Design review of the part built by this model. Coordinates are the model's own, in mm. Face numbers are marked on the shaded views. A direction names the side the tool comes from. Coordinates: 2 decimals unless noted, no trailing zeros. Write each loop counter-clockwise with the first axis right and the second up, starting at its lowest first coordinate (ties: lowest second). Pieces come first, ordered by that corner, then holes.
Q1. Insertion check: pin 1 (4 mm diameter, centred on x = -7, z = -7.5, fed in from +Y); pin 2 (1 mm diameter, centred on x = -11.5, z = -11.5, fed in from +Y); pin 3 (1.7 mm diameter, centred on x = 0, z = 0.5, fed in from +Y). Each pin has a flat end and moves straight along its axis. Give the tip position at first contact, or say it passes through.
Q2. For probe 1 along X at (y, z) = (23.75, 11.43) (3 decimals); probe 2 along X at (y, z) = (8, -0.25); probe 3 along Z at (x, y) = (-0.5, 23), list the stretches that pass through material, from the lowest coordinate up.
Q3. Take a section at A-A (y = 4). Give the boundary of the cut face in (x, z) (1 decimal).
Q4. Mouldability with a two-part tool opening along Z and no side actions: class the marked faces 3, 4 and 5 as pulls with the +Z half, pulls with the -Z half, needs draft (parallel to the pull), parting line crosses it, or undercut.
Q5. Take a section at D-D (y = 21.5). Give the boundary of the cut face in (x, z) (3 decimals).
Q6. Take a section at B-B (z = 9.5). Give the boundary of the cut face in (x, y).
Q7. Machinability: for the marked faces 1 and 2, which of the approach directions +Z, -Z, +X, -X, +Y, -Y give a long, thin tool a straight path to every point of the face, cutting with its end or side? Answer none if there is none.
Q8. Take a section at C-C (x = -11.43). Give the boundary of the cut face in (y, z) (3 decimals), and give its area (3 significant figures).
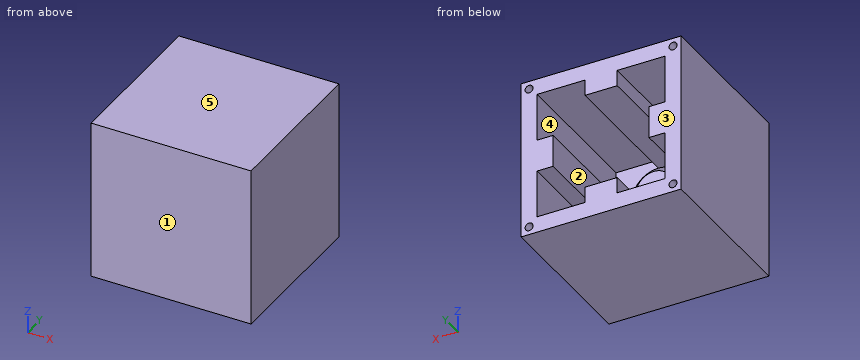
```python
from build123d import *

# Parameters (mm, degrees)
SKETCH1_W           = 25.4
SKETCH1_H           = 25.4
BOSS_EXTRUDE1_DEPTH = 25.4
CUT_EXTRUDE2_DEPTH  = 22.86
SKETCH4_R           = 0.635
CUT_EXTRUDE4_DEPTH  = 7.62
SKETCH5_R           = 4.1275
BOSS_EXTRUDE2_DEPTH = 7.62
CHAMFER1_SIZE       = 1.27


with BuildPart() as part:
    # Sketch1 → Boss-Extrude1 (new body)
    with BuildSketch(Plane(origin=(0, 0, 0), x_dir=(1, 0, 0), z_dir=(0, 1, 0))):
        Rectangle(SKETCH1_W, SKETCH1_H)
    extrude(amount=BOSS_EXTRUDE1_DEPTH)

    # Sketch3 → Cut-Extrude2 (cut)
    with BuildSketch(Plane(origin=(0, 25.4, 0), x_dir=(1, 0, 0), z_dir=(0, 1, 0))):
        Polygon((10.16, 2.565122784), (7.62, 2.565122784), (7.62, -2.565122784), (10.16, -2.565122784), (10.16, -10.16), (2.565122784, -10.16), (2.565122784, -7.62), (-2.565122784, -7.62), (-2.565122784, -10.16), (-10.16, -10.16), (-10.16, -2.565122784), (-7.62, -2.565122784), (-7.62, 2.565122784), (-10.16, 2.565122784), (-10.16, 10.16), (-2.565122784, 10.16), (-2.565122784, 7.62), (2.565122784, 7.62), (2.565122784, 10.16), (10.16, 10.16), align=None)
    extrude(amount=-CUT_EXTRUDE2_DEPTH, mode=Mode.SUBTRACT)

    # Sketch4 → Cut-Extrude4 (cut)
    with BuildSketch(Plane(origin=(0, 25.4, 0), x_dir=(1, 0, 0), z_dir=(0, 1, 0))):
        with Locations(Location((11.43, 11.43, 0), (0, 0, 270))):
            Circle(SKETCH4_R)
        with Locations(Location((11.43, -11.43, 0), (0, 0, 270))):
            Circle(SKETCH4_R)
        with Locations(Location((-11.43, -11.43, 0), (0, 0, 270))):
            Circle(SKETCH4_R)
        with Locations(Location((-11.43, 11.43, 0), (0, 0, 270))):
            Circle(SKETCH4_R)
    extrude(amount=-CUT_EXTRUDE4_DEPTH, mode=Mode.SUBTRACT)

    # Sketch5 → Boss-Extrude2 (add)
    with BuildSketch(Plane(origin=(0, 2.54, 0), x_dir=(1, 0, 0), z_dir=(0, 1, 0))):
        with Locations(Location((0, 0, 0), (0, 0, 90))):
            Circle(SKETCH5_R)
    extrude(amount=BOSS_EXTRUDE2_DEPTH)

    # Chamfer1
    chamfer1_edges = [part.edges().sort_by_distance(p)[0] for p in [
        (0, 10.16, 4.1275),
    ]]
    chamfer(chamfer1_edges, length=CHAMFER1_SIZE)


solid = part.part
```
Response:
1. pin 1: stops at y = 2.54
1. pin 2: stops at y = 17.78
1. pin 3: stops at y = 10.16
2. probe 1: x = -12.7 to -12.065, -10.795 to 10.795, 12.065 to 12.7
2. probe 2: x = -12.7 to -7.62, -4.12 to 4.12, 7.62 to 12.7
2. probe 3: z = -12.7 to -7.62, 7.62 to 12.7
3. outline: (-12.7, -12.7) - (12.7, -12.7) - (12.7, 12.7) - (-12.7, 12.7) - close; circle Ø8.3 at (0, 0); hole (-10.2, -10.2) - (-2.6, -10.2) - (-2.6, -7.6) - (2.6, -7.6) - (2.6, -10.2) - (10.2, -10.2) - (10.2, -2.6) - (7.6, -2.6) - (7.6, 2.6) - (10.2, 2.6) - (10.2, 10.2) - (2.6, 10.2) - (2.6, 7.6) - (-2.6, 7.6) - (-2.6, 10.2) - (-10.2, 10.2) - (-10.2, 2.6) - (-7.6, 2.6) - (-7.6, -2.6) - (-10.2, -2.6) - close
4. face 3: needs draft
4. face 4: undercut
4. face 5: pulls with the +Z half
5. outline: (-12.7, -12.7) - (12.7, -12.7) - (12.7, 12.7) - (-12.7, 12.7) - close; hole circle Ø1.27 at (-11.43, -11.43); hole circle Ø1.27 at (-11.43, 11.43); hole (-10.16, -10.16) - (-2.565, -10.16) - (-2.565, -7.62) - (2.565, -7.62) - (2.565, -10.16) - (10.16, -10.16) - (10.16, -2.565) - (7.62, -2.565) - (7.62, 2.565) - (10.16, 2.565) - (10.16, 10.16) - (2.565, 10.16) - (2.565, 7.62) - (-2.565, 7.62) - (-2.565, 10.16) - (-10.16, 10.16) - (-10.16, 2.565) - (-7.62, 2.565) - (-7.62, -2.565) - (-10.16, -2.565) - close; hole circle Ø1.27 at (11.43, -11.43); hole circle Ø1.27 at (11.43, 11.43)
6. outline: (-12.7, 0) - (12.7, 0) - (12.7, 25.4) - (10.16, 25.4) - (10.16, 2.54) - (2.57, 2.54) - (2.57, 25.4) - (-2.57, 25.4) - (-2.57, 2.54) - (-10.16, 2.54) - (-10.16, 25.4) - (-12.7, 25.4) - close
7. face 1: +Z, -Z, +X, -X, -Y
7. face 2: +Y
8. outline: (0, -12.7) - (25.4, -12.7) - (25.4, -12.065) - (17.78, -12.065) - (17.78, -10.795) - (25.4, -10.795) - (25.4, 10.795) - (17.78, 10.795) - (17.78, 12.065) - (25.4, 12.065) - (25.4, 12.7) - (0, 12.7) - close
8. area: 626 mm2
